Autodesk Inventor part; units mm, degrees
ref_plane "YZ Plane" through (0, 0, 0) normal (1, 0, 0) x (0, 1, 0)
ref_plane "XZ Plane" through (0, 0, 0) normal (0, 1, 0) x (-1, 0, 0)
ref_plane "XY Plane" through (0, 0, 0) normal (0, 0, 1) x (1, 0, 0)
sketch "Sketch1" plane through (0, 0, 0) normal (1, 0, 0) x (0, 1, 0)
  circle A0 centre (0, 0) radius 50
  line L0 (-36.9504, -64) -> (-73.9008, 0)
  line L1 (-73.9008, 0) -> (-36.9504, 64)
  line L2 (-36.9504, 64) -> (36.9504, 64)
  line L3 (36.9504, 64) -> (73.9008, 0)
  line L4 (73.9008, 0) -> (36.9504, -64)
  line L5 (36.9504, -64) -> (-36.9504, -64)
  dimension "d0" = 100
  dimension "d1" = 64
extrude "Extrusion1" add sketch "Sketch1" along normal mid plane 110
sketch "Sketch3" plane through (0, 0, 0) normal (1, 0, 0) x (0, 1, 0)
  line L0 (-43.3013, -75) -> (-86.6025, 0)
  line L1 (-86.6025, 0) -> (-43.3013, 75)
  line L2 (-43.3013, 75) -> (43.3013, 75)
  line L3 (43.3013, 75) -> (86.6025, 0)
  line L4 (86.6025, 0) -> (43.3013, -75)
  line L5 (43.3013, -75) -> (-43.3013, -75)
  circle A0 centre (0, 0) radius 50
  dimension "d4" = 75
extrude "Extrusion2" add sketch "Sketch3" along normal mid plane 50
thread "Thread1"
properties part number "uniao assento conico 4 inch"
The model under review builds one solid part; all positions refer to its coordinate system, in mm. A direction names the side the tool comes from. Round coordinates to 2 decimals unless told otherwise and drop trailing zeros. Write each loop counter-clockwise with the first axis right and the second up, starting at its lowest first coordinate (ties: lowest second). Pieces come first, ordered by that corner, then holes. Notation, with made-up numbers: M -4.5,35.25 L 32.5,35.25 A20 ccw 32.5,72.25 Z; hole C 2.5,74 d3. An arc over 180 degrees is marked long. Use a Markdown table: item, result. Add a question column.
Q1. Machinability: for faces 1 (the face through (39.79, -55.167, -32.448)), 2 (the face through (-40, -1, 64)), 3 (the face through (-40.21, -55.684, 31.552)), 4 (the face through (40, -1, 64)), which of the approach directions +Z, -Z, +X, -X, +Y, -Y give a long, thin tool a straight path to every point of the face, cutting with its end or side? Answer none if there is none.
Q2. Insertion check: pin 1 (24 mm diameter, centred on x = -33.5, y = 2, fed in from +Z); pin 2 (3 mm diameter, centred on x = -18.5, z = 58, fed in from +Y); pin 3 (8 mm diameter, centred on x = 26, z = -37, fed in from -Y); pin 4 (1.5 mm diameter, centred on x = -39.5, y = 41, fed in from -Z). Each pin has a flat end and moves straight along its axis. Give the tip position at first contact, or say it passes through.
Q3. We need section C-C, the plane y = 68. State the section outline as (x, z) points, plus the area to 3 significant figures.
Q4. We need section B-B, the plane z = -21.5. State the section outline as (x, y) points.
Q5. We need section A-A, the plane y = 0. State the section outline as (x, z) points.
Q6. To check wall thickness, follow line 1 (Z direction, x = -3, y = 0); line 2 (Y direction, x = 38.5, z = 32); line 3 (Y direction, x = 19, z = -22). State the ranges of each line that lie inside material, in increasing order.
Findings below:
| question | item | result |
|---|---|---|
| 1 | face 1 | -Z, +X, -Y |
| 1 | face 2 | +Z, -X, +Y, -Y |
| 1 | face 3 | +Z, -X, -Y |
| 1 | face 4 | +Z, +X, +Y, -Y |
| 2 | pin 1 | stops at z = 75 |
| 2 | pin 2 | stops at y = 53.98 |
| 2 | pin 3 | stops at y = -67.48 |
| 2 | pin 4 | stops at z = -58.28 |
| 3 | outline | M -55,-10.22 L -25,-10.22 L -25,-32.22 L 25,-32.22 L 25,-10.22 L 55,-10.22 L 55,10.22 L 25,10.22 L 25,32.22 L -25,32.22 L -25,10.22 L -55,10.22 Z |
| 3 | area | 4,450 mm² |
| 4 | outline | M -55,-61.49 L -25,-61.49 L -25,-74.19 L 25,-74.19 L 25,-61.49 L 55,-61.49 L 55,-45.14 L -55,-45.14 Z; M -55,45.14 L 55,45.14 L 55,61.49 L 25,61.49 L 25,74.19 L -25,74.19 L -25,61.49 L -55,61.49 Z |
| 5 | outline | M -55,-64 L -25,-64 L -25,-75 L 25,-75 L 25,-64 L 55,-64 L 55,-50 L -55,-50 Z; M -55,50 L 55,50 L 55,64 L 25,64 L 25,75 L -25,75 L -25,64 L -55,64 Z |
| 6 | line 1 | z = -75 to -50, 50 to 75 |
| 6 | line 2 | y = -55.43 to -38.42, 38.42 to 55.43 |
| 6 | line 3 | y = -73.9 to -44.9, 44.9 to 73.9 |
